CAD build for the part. Positions are in the model's coordinates, mm. Coordinates: 2 decimals unless noted, no trailing zeros. Order: outer loops, then holes, each group sorted by start corner. A loop starts at its lowest first (then second) coordinate and runs counter-clockwise, first axis right, second up. Notation, with made-up numbers: (-5, 23) - (17, 23) arc R23 cw to (17, 31) - close; hole circle Ø1 at (26.5, 14). An arc over 180 degrees is marked (long way). Return JSON: item names as keys, results as strings.
Autodesk Inventor part; units mm, degrees
ref_plane "YZ Plane" through (0, 0, 0) normal (1, 0, 0) x (0, 1, 0)
ref_plane "XZ Plane" through (0, 0, 0) normal (0, 1, 0) x (-1, 0, 0)
ref_plane "XY Plane" through (0, 0, 0) normal (0, 0, 1) x (1, 0, 0)
sketch "Sketch1" plane through (0, 0, 0) normal (0, 1, 0) x (-1, 0, 0)
  circle A0 centre (0, 0) radius 15
  line L0 (0, -15) -> (0, -19)
  line L1 (0, -19) -> (2.5, -19)
  line L2 (2.5, -19) -> (2.5, -14.7902)
  line L3 (0, -19) -> (-2.5, -19)
  line L4 (-2.5, -19) -> (-2.5, -14.7902)
  line L5 (6.6169, 0) -> (-6.6879, 0)
  line L6 (0, 15) -> (0, 19)
  line L7 (0, 19) -> (2.5, 19)
  line L8 (2.5, 19) -> (2.5, 14.7902)
  line L9 (0, 19) -> (-2.5, 19)
  line L10 (-2.5, 19) -> (-2.5, 14.7902)
  point P0 (2.5, 14.7902)
  point P1 (-2.5, 14.7902)
  dimension "d0" = 4
  dimension "d1" = 2.5
  dimension "d13" = 30
extrude "Extrusion1" add sketch "Sketch1" along normal blind 6
sketch "Sketch2" plane through (0, 6, 0) normal (0, 1, 0) x (1, 0, 0)
  circle A0 centre (2.0473, 7.2692) radius 2.5
  circle A1 centre (2.0473, 7.2692) radius 5 construction
  circle A2 centre (6.8395, 8.6957) radius 1.5
  circle A3 centre (2.0473, 7.2692) radius 5 construction
  circle A4 centre (0.6208, 12.0614) radius 1.5
  circle A5 centre (2.0473, 7.2692) radius 5 construction
  circle A6 centre (-2.7449, 5.8427) radius 1.5
  circle A7 centre (2.0473, 7.2692) radius 5 construction
  circle A8 centre (3.4738, 2.477) radius 1.5
  circle A9 centre (-6.6513, -1.8166) radius 2.5
  circle A10 centre (-6.6513, -1.8166) radius 5 construction
  circle A11 centre (-9.5082, 2.2868) radius 1.5
  circle A12 centre (-6.6513, -1.8166) radius 5 construction
  circle A13 centre (-10.7547, -4.6735) radius 1.5
  circle A14 centre (-6.6513, -1.8166) radius 5 construction
  circle A15 centre (-3.7944, -5.92) radius 1.5
  circle A16 centre (-6.6513, -1.8166) radius 5 construction
  circle A17 centre (-2.5478, 1.0403) radius 1.5
  circle A18 centre (5.3395, -5.0913) radius 2.5
  circle A19 centre (5.3395, -5.0913) radius 5 construction
  circle A20 centre (2.0648, -8.8697) radius 1.5
  circle A21 centre (5.3395, -5.0913) radius 5 construction
  circle A22 centre (9.1179, -8.3659) radius 1.5
  circle A23 centre (5.3395, -5.0913) radius 5 construction
  circle A24 centre (8.6142, -1.3128) radius 1.5
  circle A25 centre (5.3395, -5.0913) radius 5 construction
  circle A26 centre (1.5611, -1.8166) radius 1.5
  circle A27 centre (-8.7734, 7.2692) radius 2.5
  circle A28 centre (9.859, 3.1889) radius 2.5
  circle A29 centre (-4.0478, -10.8701) radius 2.1836
  dimension "d17" = 10
  dimension "d23" = 10
  dimension "d35" = 10
  dimension "d16" = 5
  dimension "d18" = 3
  dimension "d19" = 360
  dimension "d22" = 5
  dimension "d24" = 3
  dimension "d25" = 360
  dimension "d34" = 5
  dimension "d36" = 3
  dimension "d37" = 360
  dimension "d38" = 5
  dimension "d39" = 5
extrude "Extrusion2" cut sketch "Sketch2" against normal blind 5
sketch "Sketch3" plane through (0, 6, 0) normal (0, 1, 0) x (1, 0, 0)
  point P0 (0, 0)
properties part number "joy stick part 1"
Item 1: Band-saw the part on C-C, the plane z = 5.5. List the corners of the cut face in (x, y), then the cut area to 3 significant figures.
Findings below:
{"outline": "(-13.96, 0) - (13.96, 0) - (13.96, 6) - (7.81, 6) - (7.81, 1) - (2.87, 1) - (2.87, 6) - (-2.35, 6) - (-2.35, 1) - (-5.23, 1) - (-5.23, 6) - (-9.5, 6) - (-9.5, 1) - (-12.01, 1) - (-12.01, 6) - (-13.96, 6) - close", "area": "116 mm²"}
Item 2: Drop flat-ended pins along their axis: P1, Ø4.5, axis at x = 2.05, z = -7.27, coming from the +Y side; P2, Ø3.5, axis at y = 2, z = 17.5, coming from the -X side; P3, Ø1.3, axis at y = 3.5, z = -17, coming from the +X side. Give the stop position or say it passes through.
Findings below:
{"P1": "stops at y = 1", "P2": "stops at x = -2.5", "P3": "stops at x = 2.5"}
Item 3: Band-saw the part on A-A, the plane y = 4.2. Count the separate pieces of the cut face and the enclosed holes in it, then the cut area to 3 significant figures.
Findings below:
{"separate pieces": "1", "enclosed holes": "18", "area": "550 mm²"}
Item 4: Mould opens along X. For faces 1 (the flat face through (0, 3, 19)), 2 (the cylindrical face through (15, 3, 0)), 3 (the cylindrical face through (7.51, 3.54, 0.3)) say: released by +X, released by -X, zero draft, split by the parting line, or undercut.
Findings below:
{"face 1": "zero draft", "face 2": "released by +X", "face 3": "undercut"}
Item 5: Band-saw the part on B-B, the plane x = -6.75. List the corners of the cut face in (y, z), then the cut area to 3 significant figures.
Findings below:
{"outline": "(0, -13.4) - (6, -13.4) - (6, -8.74) - (1, -8.74) - (1, -5.8) - (6, -5.8) - (6, -0.68) - (1, -0.68) - (1, 4.31) - (6, 4.31) - (6, 13.4) - (0, 13.4) - close", "area": "121 mm²"}
Item 6: Band-saw the part on D-D, the plane x = 9.25. List the corners of the cut face in (y, z).
Findings below:
{"outline": "(0, -11.81) - (6, -11.81) - (6, -5.61) - (1, -5.61) - (1, -0.76) - (6, -0.76) - (6, -0.05) - (1, -0.05) - (1, 2.67) - (6, 2.67) - (6, 6.87) - (1, 6.87) - (1, 9.86) - (6, 9.86) - (6, 11.81) - (0, 11.81) - close"}
Item 7: Wall check: L1, parallel to Z at x = -7.75, y = 4.3; L2, parallel to Z at x = -3.25, y = 1.3; L3, parallel to Z at x = 3.75, y = 3.85. Give the ranges that are in metal, low to high. Write a range as [from, to].
Findings below:
{"L1": "z = [-12.84, -9.55], [-4.99, -0.43], [4.06, 12.84]", "L2": "z = [-14.64, -7.26], [-4.43, -2.37], [0.29, 4.52], [7.32, 8.84], [12.9, 14.64]", "L3": "z = [-14.52, -9.1], [-5.44, -3.95], [-1, 3.16], [7.02, 14.52]"}
